Part model, mm, in its own coordinate system. A direction names the side the tool comes from. Give positions to 0.01 mm unless a question says otherwise; leave off trailing zeros. Write each loop counter-clockwise with the first axis right and the second up, starting at its lowest first coordinate (ties: lowest second). Pieces come first, ordered by that corner, then holes. Notation, with made-up numbers: M 86.5,-26.5 L 90.5,-26.5 A19 cw 90.5,-8.5 Z; hole C 44.5,32.25 d9. An arc over 180 degrees is marked long. Use a Markdown table: item, result. Add a question column.
from build123d import *

# Parameters (mm, degrees)
SKETCH1_W           = 70.1
SKETCH1_H           = 37.59
BOSS_EXTRUDE1_DEPTH = 38.1
FILLET1_R           = 5
SKETCH2_W           = 12
SKETCH2_H           = 4
BOSS_EXTRUDE2_DEPTH = 5


with BuildPart() as part:
    # Sketch1 → Boss-Extrude1 (new body)
    with BuildSketch(Plane.XY):
        with Locations((6.077190332, 7.269320242)):
            Rectangle(SKETCH1_W, SKETCH1_H)
    extrude(amount=BOSS_EXTRUDE1_DEPTH)

    # Fillet1
    fillet1_edges = [part.edges().sort_by_distance(p)[0] for p in [
        (6.077190332, -11.525679758, 38.1),
        (41.127190332, 7.269320242, 38.1),
        (6.077190332, 26.064320242, 38.1),
        (41.127190332, 7.269320242, 0),
        (6.077190332, -11.525679758, 0),
        (-28.972809668, 7.269320242, 0),
        (6.077190332, 26.064320242, 0),
        (-28.972809668, 7.269320242, 38.1),
        (41.127190332, 26.064320242, 19.05),
        (41.127190332, -11.525679758, 19.05),
        (-28.972809668, -11.525679758, 19.05),
        (-28.972809668, 26.064320242, 19.05),
    ]]
    fillet(fillet1_edges, radius=FILLET1_R)

    # Sketch2 → Boss-Extrude2 (add)
    with BuildSketch(Plane(origin=(0, 26.064320242, 0), x_dir=(1, 0, 0), z_dir=(0, 1, 0))):
        with Locations((-17.972809668, -13)):
            Rectangle(SKETCH2_W, SKETCH2_H)
        with Locations((-17.972809668, -7)):
            Rectangle(SKETCH2_W, SKETCH2_H)
    extrude(amount=BOSS_EXTRUDE2_DEPTH)


solid = part.part
1. Flat gauge pins, fed straight in: pin 1 (8 mm diameter, centred on x = -13.5, z = 19.5, fed in from +Y); pin 2 (3 mm diameter, centred on y = 28.5, z = 13, fed in from -X); pin 3 (4 mm diameter, centred on x = 11.5, y = 26.5, fed in from +Z); pin 4 (2 mm diameter, centred on x = 4.5, y = 22, fed in from +Z). Where does each tip first touch, or does it go through?
2. Cut at D-D (x = -13.5). Write the cut outline in (y, z), then the cut area to 3 significant figures.
3. Drill centre lines: probe 1 along Y at (x, z) = (6, 17); probe 2 along X at (y, z) = (26.5, 13.5); probe 3 along Y at (x, z) = (11, 33.5). Where is each one in solid material? Low to high. Write a range as [from, to].
4. Cut at A-A (z = 8). Write the cut outline in (x, y).
5. Cut at C-C (y = 23.5). Write the cut outline in (x, z).
6. Tool access for faces 1 (the flat face through (-23.973, 29, 13)), 2 (the flat face through (-18, 29, 5)), 3 (the cylindrical face through (6.498, -10.1, 1.504)), 4 (the flat face through (-18, 29, 15)): list every direction of +Z, -Z, +X, -X, +Y, -Y with a clear straight run to the whole face (end or side of a thin tool).
7. Cut at B-B (x = 0). Write the cut outline in (y, z), then the cut area to 3 significant figures.
A:
| question | item | result |
|---|---|---|
| 1 | pin 1 | stops at y = 26.06 |
| 1 | pin 2 | stops at x = -23.97 |
| 1 | pin 3 | stops at z = 36.73 |
| 1 | pin 4 | stops at z = 38.1 |
| 2 | outline | M -11.53,5 A5 ccw -6.53,0 L 21.06,0 A5 ccw 26.06,5 L 31.06,5 L 31.06,9 L 26.06,9 L 26.06,11 L 31.06,11 L 31.06,15 L 26.06,15 L 26.06,33.1 A5 ccw 21.06,38.1 L -6.53,38.1 A5 ccw -11.53,33.1 Z |
| 2 | area | 1,450 mm² |
| 3 | probe 1 | y = [-11.53, 26.06] |
| 3 | probe 2 | x = [-23.97, -11.97] |
| 3 | probe 3 | y = [-11.51, 26.05] |
| 4 | outline | M -28.97,-6.53 A5 ccw -23.97,-11.53 L 36.13,-11.53 A5 ccw 41.13,-6.53 L 41.13,21.06 A5 ccw 36.13,26.06 L -11.97,26.06 L -11.97,31.06 L -23.97,31.06 L -23.97,26.06 A5 ccw -28.97,21.06 Z |
| 5 | outline | M -28.34,5 A4.37 ccw -23.97,0.63 L 36.13,0.63 A4.37 ccw 40.49,5 L 40.49,33.1 A4.37 ccw 36.13,37.47 L -23.97,37.47 A4.37 ccw -28.34,33.1 Z |
| 6 | face 1 | +Z, -Z, -X, +Y |
| 6 | face 2 | -Z, +X, -X, +Y |
| 6 | face 3 | -Z, +X, -X, -Y |
| 6 | face 4 | +Z, +X, -X, +Y |
| 7 | outline | M -11.53,5 A5 ccw -6.53,0 L 21.06,0 A5 ccw 26.06,5 L 26.06,33.1 A5 ccw 21.06,38.1 L -6.53,38.1 A5 ccw -11.53,33.1 Z |
| 7 | area | 1,410 mm² |
